For this review, use the dimensioned drawing (mm, ordinates from the lowest corner) and the shaded views. Coordinates: 2 decimals unless noted, no trailing zeros. Write each loop counter-clockwise with the first axis right and the second up, starting at its lowest first coordinate (ties: lowest second). Pieces come first, ordered by that corner, then holes.
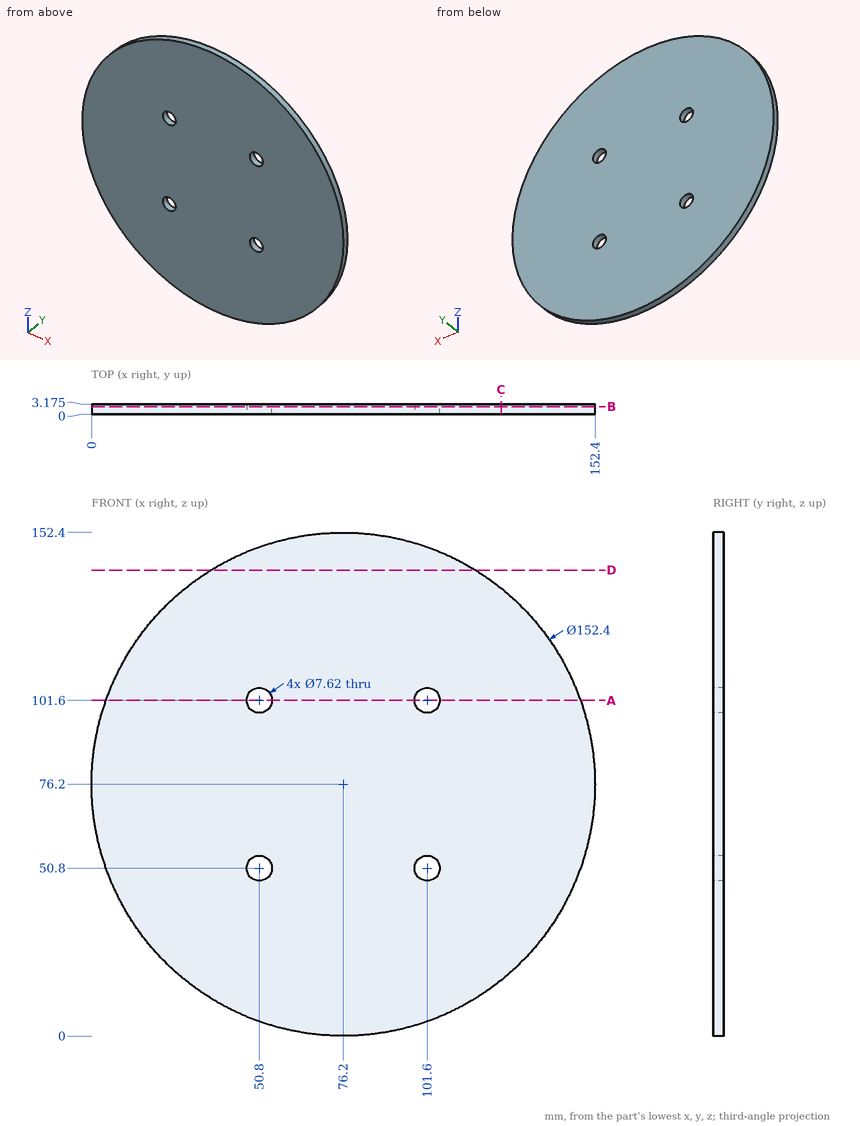
(1) Consider section D-D (z = 141). Give the boundary of the cut face in (x, y) (3 decimals).
(2) Wall thickness on line 1 (Z direction, x = 53.5, y = 1.05); line 2 (Z direction, x = 53, y = 0.7); line 3 (X direction, y = 1.55, z = 101.6): over which ranges is each line inside the solid? List them lowest first.
(3) Consider section A-A (z = 101.6). Give the boundary of the cut face in (x, y) (3 decimals), plus the area to 3 significant figures.
(4) Consider section B-B (y = 2.4). Give the boundary of the cut face in (x, z).
(5) Consider section C-C (x = 124). Give the boundary of the cut face in (y, z) (3 decimals).
(6) Insertion check: pin 1 Ø1 at (x, y) = (70, 0.5) entering from -Z; pin 2 Ø1 at (x, y) = (58.5, 0.5) entering from +Z. Each pin has a flat end and moves straight along its axis. Give the tip position at first contact, or say it passes through.
Results:
1. outline: (36.108, 0) - (116.292, 0) - (116.292, 3.175) - (36.108, 3.175) - close
2. line 1: z = 3.46 to 48.11, 53.49 to 98.91, 104.29 to 148.94
2. line 2: z = 3.62 to 47.69, 53.91 to 98.49, 104.71 to 148.78
2. line 3: x = 4.36 to 46.99, 54.61 to 97.79, 105.41 to 148.04
3. outline: (4.358, 0) - (46.99, 0) - (46.99, 3.175) - (4.358, 3.175) - close; (54.61, 0) - (97.79, 0) - (97.79, 3.175) - (54.61, 3.175) - close; (105.41, 0) - (148.042, 0) - (148.042, 3.175) - (105.41, 3.175) - close
3. area: 408 mm2
4. outline: circle Ø152.4 at (76.2, 76.2); hole circle Ø7.62 at (50.8, 50.8); hole circle Ø7.62 at (50.8, 101.6); hole circle Ø7.62 at (101.6, 50.8); hole circle Ø7.62 at (101.6, 101.6)
5. outline: (0, 16.857) - (3.175, 16.857) - (3.175, 135.543) - (0, 135.543) - close
6. pin 1: stops at z = 0.21
6. pin 2: stops at z = 150.43
